Verification items for the finished model (mm, model axes). A direction names the side the tool comes from. Round coordinates to 2 decimals unless told otherwise and drop trailing zeros. Write each loop counter-clockwise with the first axis right and the second up, starting at its lowest first coordinate (ties: lowest second). Pieces come first, ordered by that corner, then holes. Notation, with made-up numbers: (48.5, 78) -> (72.5, 78) arc R20 ccw to (72.5, 97) -> close; hole circle Ø1 at (72.25, -33.5). An arc over 180 degrees is marked (long way). Answer as a JSON object with one key per item and string values. Group by question number.
(1) Gauge pin test, flat ends, axial feed: pin 1 Ø3 at (x, y) = (9.5, -33.5) entering from +Z; pin 2 Ø2 at (x, y) = (4.5, -22) entering from -Z; pin 3 Ø12 at (y, z) = (-23.5, -10) entering from -X; pin 4 Ø1 at (x, z) = (7.5, 4) entering from -Y. Record the tip position at first contact, or that the pin passes through.
(2) Scan lines: L1, parallel to Y at x = 5.75, z = 5; L2, parallel to Z at x = 4.75, y = -31; L3, parallel to Z at x = 5.5, y = -37. Record each from-to range of solid material in increasing order. Write a range as from..to.
(3) Sectioned sample at B-B on x = 0. Record the cut outline in (y, z), and give its area (3 significant figures).
(4) Sectioned sample at D-D on x = -12.75. Record the cut outline in (y, z), and give its area (3 significant figures).
(5) Sectioned sample at A-A on z = 0. Record the cut outline in (x, y).
(6) Set-up check for faces 1 (the face through (0, 15, 0)), 2 (the face through (-1.31, -29.79, -5.89)): record each of +Z, -Z, +X, -X, +Y, -Y from which the full face is reachable in a straight line by a thin tool's end or side.
(7) Sectioned sample at C-C on y = -35. Record the cut outline in (x, z).
```python
from build123d import *

# Parameters (mm, degrees)
F0_W     = 30
F0_H     = 30
F1_DEPTH = 15
F2_R     = 6.035824
F3_DEPTH = 30


with BuildPart() as f1:
    # F0 (on Front) → F1 (new body, symmetric)
    with BuildSketch(Plane.XZ):
        Rectangle(F0_W, F0_H)
    extrude(amount=F1_DEPTH, both=True)

    # F2 (on face) → F3 (join)
    with BuildSketch(Plane.XZ.offset(15)):
        Circle(F2_R)
    extrude(amount=F3_DEPTH)


solid = f1.part
```
Computed values:
{
 "1": {"pin 1": "through", "pin 2": "z = -4.92", "pin 3": "x = -4.52", "pin 4": "y = -15"},
 "2": {"L1": "-15..15", "L2": "-3.72..3.72", "L3": "-2.49..2.49"},
 "3": {"outline": "(-45, -6.04) -> (-15, -6.04) -> (-15, -15) -> (15, -15) -> (15, 15) -> (-15, 15) -> (-15, 6.04) -> (-45, 6.04) -> close", "area": "1,260 mm2"},
 "4": {"outline": "(-15, -15) -> (15, -15) -> (15, 15) -> (-15, 15) -> close", "area": "900 mm2"},
 "5": {"outline": "(-15, -15) -> (-6.04, -15) -> (-6.04, -45) -> (6.04, -45) -> (6.04, -15) -> (15, -15) -> (15, 15) -> (-15, 15) -> close"},
 "6": {"face 1": "+Z, -Z, +X, -X, +Y", "face 2": "-Y"},
 "7": {"outline": "circle Ø12.07 at (0, 0)"}
}
